Geometry check sheet. Reference: the model listing, model coordinates, mm. A direction names the side the tool comes from. Coordinates: 2 decimals unless noted, no trailing zeros. Write each loop counter-clockwise with the first axis right and the second up, starting at its lowest first coordinate (ties: lowest second). Pieces come first, ordered by that corner, then holes. Notation, with made-up numbers: (20.5, -39) -> (58.5, -39) arc R16 cw to (58.5, -17) -> close; hole circle Ø1 at (21, 30.25). An arc over 180 degrees is marked (long way). Answer in a Markdown table with one row per item. Add a question column.
1. Cross-section at D-D on z = -42.5. Record the cut outline in (x, y).
2. Mould release check, pull along Z, two halves, no side actions. Record for faces 4 (the flat face through (1.972, 56.675, 64.713)), 5 (the flat face through (2, 25, 45)), 6 (the flat face through (2, 149.9, -26.4)): pulls with the +Z half, pulls with the -Z half, needs draft (parallel to the pull), parting line crosses it, or undercut.
3. Cross-section at A-A on y = 144.5. Record the cut outline in (x, z).
4. Cross-section at B-B on y = 259. Record the cut outline in (x, z), and give its area (3 significant figures).
5. Depth check by flat-ended pin: P1, Ø4.5, axis at y = 78.52, z = 18.53, coming from the +X side; P2, Ø2, axis at x = 2, z = 1.5, coming from the -Y side; P3, Ø1.5, axis at x = 3.5, z = 56, coming from the +Y side; P4, Ø1, axis at x = 1, z = -50.5, coming from the +Y side. Enter the tip coordinate at first touch or a pass-through.
6. Scan lines: L1, parallel to Y at x = 0.55, z = 7.5; L2, parallel to Z at x = 2.6, y = 187; L3, parallel to Z at x = 3.3, y = 273. Record each from-to range of solid material in increasing order. Write a range as from..to.
7. Cross-section at C-C on x = 1.3. Give the number of separate pieces and of enclosed holes in the cut face, and give its area (3 significant figures).
8. Set-up check for faces 1 (the flat face through (0, 127, 28)), 2 (the flat face through (2, 25, -45)), 3 (the flat face through (2.03, 143.57, 17.57)): record each of +Z, -Z, +X, -X, +Y, -Y from which the full face is reachable in a straight line by a thin tool's end or side.
```python
from build123d import *

# Parameters (mm, degrees)
SKETCH_1_R          = 2.7
EXTRUDE_1_DEPTH     = 4
CUT_EXTRUDE_1_REACH = 414.179
FILLET_1_R          = 3
FILLET_2_R          = 2


with BuildPart() as part:
    # 草圖1 → 填料-伸長1 (new body)
    with BuildSketch(Plane(origin=(0, 0, 0), x_dir=(0, 0, -1), z_dir=(1, 0, 0))):
        Polygon((-55, 0), (-35, 50), (35, 50), (55, 0), (93, 0), (93, 11.24256), (37.5, 100.38), (15, 200.76), (10, 251.53), (10, 401.53), (-10, 401.53), (-10, 251.53), (-15, 200.76), (-37.5, 100.38), (-93, 11.24256), (-93, 0), align=None)
        with Locations((28.317422225, 96.006946316)):
            Circle(SKETCH_1_R, mode=Mode.SUBTRACT)
        with Locations((-18.525349225, 78.521101672)):
            Circle(SKETCH_1_R, mode=Mode.SUBTRACT)
        with Locations((68, 11)):
            Circle(SKETCH_1_R, mode=Mode.SUBTRACT)
        with Locations((84, 11)):
            Circle(SKETCH_1_R, mode=Mode.SUBTRACT)
        with Locations((-84, 11)):
            Circle(SKETCH_1_R, mode=Mode.SUBTRACT)
        with Locations((-68, 11)):
            Circle(SKETCH_1_R, mode=Mode.SUBTRACT)
        with Locations((0, 186.76)):
            Circle(SKETCH_1_R, mode=Mode.SUBTRACT)
        with Locations((0, 390.53)):
            Circle(SKETCH_1_R, mode=Mode.SUBTRACT)
    extrude(amount=EXTRUDE_1_DEPTH)

    # 草圖3 → 除料-伸長1 (cut, up to next)
    with BuildSketch(Plane(origin=(4, 0, 0), x_dir=(0, 0, -1), z_dir=(1, 0, 0)), mode=Mode.PRIVATE) as cut_extrude_1_sk1:
        Polygon((-10.525924933, 175), (-25.095560318, 110), (25.095560318, 110), (10.525924933, 175), align=None)
    cut_extrude_1_tool1 = extrude(cut_extrude_1_sk1.sketch, amount=-CUT_EXTRUDE_1_REACH, mode=Mode.PRIVATE) & part.part
    add(cut_extrude_1_tool1.solids().sort_by_distance((4, 138.06903, 0))[0], mode=Mode.SUBTRACT)

    # 圓角1
    fillet_1_edges = [part.edges().sort_by_distance(p)[0] for p in [
        (2, 175, 10.525924933),
        (2, 175, -10.525924933),
        (2, 110, -25.095560318),
        (2, 110, 25.095560318),
    ]]
    fillet(fillet_1_edges, radius=FILLET_1_R)

    # 圓角2
    fillet_2_edges = [part.edges().sort_by_distance(p)[0] for p in [
        (2, 11.24256, -93),
        (2, 0, -93),
        (2, 0, -55),
        (2, 50, -35),
        (2, 50, 35),
        (2, 0, 55),
        (2, 0, 93),
        (2, 11.24256, 93),
    ]]
    fillet(fillet_2_edges, radius=FILLET_2_R)


solid = part.part
```
Results found:
| question | item | result |
|---|---|---|
| 1 | outline | (0, 31.25) -> (4, 31.25) -> (4, 92.35) -> (0, 92.35) -> close |
| 2 | face 4 | pulls with the +Z half |
| 2 | face 5 | undercut |
| 2 | face 6 | pulls with the -Z half |
| 3 | outline | (0, -27.61) -> (4, -27.61) -> (4, -17.36) -> (0, -17.36) -> close; (0, 17.36) -> (4, 17.36) -> (4, 27.61) -> (0, 27.61) -> close |
| 4 | outline | (0, -10) -> (4, -10) -> (4, 10) -> (0, 10) -> close |
| 4 | area | 80.0 mm^2 |
| 5 | P1 | passes through |
| 5 | P2 | stops at y = 50 |
| 5 | P3 | stops at y = 71.87 |
| 5 | P4 | stops at y = 80.3 |
| 6 | L1 | y = 50..110, 175..401.53 |
| 6 | L2 | z = -18.08..-2.69, 2.69..18.08 |
| 6 | L3 | z = -10..10 |
| 7 | separate pieces | 1 |
| 7 | enclosed holes | 9 |
| 7 | area | 16,300 mm^2 |
| 8 | face 1 | +Z, -Z, -X, +Y, -Y |
| 8 | face 2 | +X, -X, -Y |
| 8 | face 3 | +X, -X |
